Build history of the part. All positions in model axes, mm. A direction names the side the tool comes from. Coordinates: 2 decimals unless noted, no trailing zeros. Loops run counter-clockwise (first coordinate to the right, second up) from the corner with the lowest first, then second, coordinate; pieces in that order, holes last.
(1) Two-plate mould, pull along X, no slides. Class faces 1 (the face through (27.006, -100.787, 9.86)), 2 (the face through (71, 20, 73)), 3 (the face through (29.7, 17, 99.8)), 4 (the face through (97, -34, 20)): pulls with the +X half, pulls with the -X half, needs draft (parallel to the pull), parting line crosses it, or undercut.
(2) Slice it at D-D (x = -12). Give the cut face in (y, z).
(3) Wall check: L1, parallel to Y at x = 30.5, z = 8; L2, parallel to X at y = -66.5, z = 34.5; L3, parallel to Y at x = 60, z = 50. Give the ranges that are in metal, low to high.
(4) Slice it at B-B (z = 66). Give the cut face in (x, y).
(5) Slice it at C-C (y = 4). Give the cut face in (x, z).
(6) Flat gauge pins, fed straight in: P1, Ø4, axis at x = 13.5, y = -91.5, coming from the +Z side; P2, Ø12, axis at y = -99.5, z = 17, coming from the -X side; P3, Ø2, axis at y = -29, z = 31.5, coming from the -X side. Where does each tip first touch, or does it go through?
(7) Slice it at A-A (y = -15). Give the cut face in (x, z).
(8) Tool access for faces 5 (the face through (55.25, -88.42, 4.93)), 6 (the face through (103.73, -10.48, 14.93)), 7 (the face through (26.984, 4.93, 100.705)): list every direction of +Z, -Z, +X, -X, +Y, -Y with a clear straight run to the whole face (end or side of a thin tool).
from build123d import *

# Parameters (mm, degrees)
F1_ANGLE  = 90
F3_DEPTH  = 20
F5_DEPTH  = 20
F7_DEPTH  = 20
F8_R      = 10
F11_DEPTH = 10


with BuildPart() as f1:
    # F0 (on Right) → F1 (revolve)
    with BuildSketch(Plane.YZ):
        with BuildLine():
            Line((0, 94.3), (0, 114.3))
            ThreePointArc((0, 114.3), (-80.8223050896, 80.8223050896), (-114.3, 0))
            Line((-114.3, 0), (-94.3, 0))
            ThreePointArc((-94.3, 0), (-66.6801694659, 66.6801694659), (0, 94.3))
        make_face()
    revolve(axis=Axis((0, 0, 104.3), (0, 0, 1)), revolution_arc=F1_ANGLE)

    # F2 (on face) → F3 (join)
    with BuildSketch(Plane(origin=(0, 0, 0), x_dir=(-1, 0, 0), z_dir=(0, 1, 0))):
        with BuildLine():
            Line((-26.2183692689, 97.8482862031), (-27.7712835395, 103.6438411608))
            ThreePointArc((-27.7712835395, 103.6438411608), (-75.8725576213, 75.8725576213), (-103.6438411608, 27.7712835395))
            Line((-103.6438411608, 27.7712835395), (-97.8482862031, 26.2183692689))
            ThreePointArc((-97.8482862031, 26.2183692689), (-71.6299169342, 71.6299169342), (-26.2183692689, 97.8482862031))
        make_face()
    extrude(amount=F3_DEPTH)

    # F4 (on face) → F5 (join)
    with BuildSketch(Plane.YZ):
        with BuildLine():
            ThreePointArc((-97.8482862031, 26.2183692689), (-71.6299169342, 71.6299169342), (-26.2183692689, 97.8482862031))
            Line((-26.2183692689, 97.8482862031), (-27.7712835395, 103.6438411608))
            ThreePointArc((-27.7712835395, 103.6438411608), (-75.8725576213, 75.8725576213), (-103.6438411608, 27.7712835395))
            Line((-103.6438411608, 27.7712835395), (-97.8482862031, 26.2183692689))
        make_face()
    extrude(amount=-F5_DEPTH)

    # F6 (on face) → F7 (cut)
    with BuildSketch(Plane(origin=(0, 0, 0), x_dir=(1, 0, 0), z_dir=(0, 0, -1))):
        with BuildLine():
            Line((27.7712835395, 103.6438411608), (26.2183692689, 97.8482862031))
            ThreePointArc((26.2183692689, 97.8482862031), (40.3932806821, 92.8981855352), (53.6808214668, 85.9072721406))
            Line((53.6808214668, 85.9072721406), (56.8603370522, 90.9955607176))
            ThreePointArc((56.8603370522, 90.9955607176), (42.7857750957, 98.4005459815), (27.7712835395, 103.6438411608))
        make_face()
        with BuildLine():
            ThreePointArc((84.9573285329, 55.171934247), (92.1790767398, 42.0084254811), (97.3758097986, 27.9220641443))
            Line((97.3758097986, 27.9220641443), (103.1433799742, 29.5758882792))
            ThreePointArc((103.1433799742, 29.5758882792), (97.6388443651, 44.496584937), (89.9893519405, 58.4397684571))
            Line((89.9893519405, 58.4397684571), (84.9573285329, 55.171934247))
        make_face()
    extrude(amount=-F7_DEPTH, mode=Mode.SUBTRACT)

    # F8
    f8_edges = [f1.edges().sort_by_distance(p)[0] for p in [
        (100.746064, 20, 26.994826),
        (26.994826, 20, 100.746064),
        (-20, -26.994826, 100.746064),
        (-20, -100.746064, 26.994826),
    ]]
    fillet(f8_edges, radius=F8_R)

    # F10 (on offset) → F11 (cut)
    with BuildSketch(Plane(origin=(0, 0, 10), x_dir=(1, 0, 0), z_dir=(0, 0, -1))):
        with BuildLine():
            ThreePointArc((97.3758097986, 27.9220641443), (99.4762319066, 19.1355503099), (100.7854867979, 10.1968451452))
            Line((100.7854867979, 10.1968451452), (106.7579299629, 10.7719260129))
            ThreePointArc((106.7579299629, 10.7719260129), (105.3709505868, 20.2546975401), (103.1433799742, 29.5758882792))
            Line((103.1433799742, 29.5758882792), (97.3758097986, 27.9220641443))
        make_face()
        Polygon((0.327321584, 0.5238240331), (0, 0), (0.4947707785, 0.5399475566), align=None)
        Polygon((0.4947707785, 0.5399475566), (0, 0), (2.5848787999, 0.7412020686), align=None)
        with BuildLine():
            Line((56.8603370522, 90.9955607176), (53.6808214668, 85.9072721406))
            ThreePointArc((53.6808214668, 85.9072721406), (61.3162809887, 80.6350028568), (68.4372880315, 74.6861942189))
            Line((68.4372880315, 74.6861942189), (72.4908292772, 79.1098582397))
            ThreePointArc((72.4908292772, 79.1098582397), (64.948044917, 85.411014872), (56.8603370522, 90.9955607176))
        make_face()
    extrude(amount=-F11_DEPTH, mode=Mode.SUBTRACT)


solid = f1.part
Response values:
1. face 1: undercut
1. face 2: needs draft
1. face 3: pulls with the -X half
1. face 4: undercut
2. outline: (-103.59, 27.97) - (-97.8, 26.41) arc R101.3 cw to (-26.41, 97.8) - (-27.97, 103.59) arc R107.3 ccw to start
3. L1: y = -109.86 to -102.87, -96.6 to -88.87
3. L2: x = 57.27 to 86.32
3. L3: y = -83.45 to -52.84
4. outline: (-20, -84.6) - (0, -84.6) - (0, -93.32) arc R93.32 ccw to (93.32, 0) - (84.6, 0) - (84.6, 20) - (76.85, 20) - (76.85, 0) - (67.35, 0) arc R67.35 cw to (0, -67.35) - (0, -76.85) - (-20, -76.85) - close
5. outline: (26.22, 97.85) arc R101.3 cw to (97.85, 26.22) - (103.64, 27.77) arc R107.3 ccw to (27.77, 103.64) - close
6. P1: stops at z = 69.83
6. P2: stops at x = 0
6. P3: stops at x = 83.5
7. outline: (0, 93.1) arc R93.1 cw to (93.1, 0) - (113.31, 0) arc R113.31 ccw to (0, 113.31) - close; hole (100.18, 10) - (106.25, 10) - (106.25, 20) - (100.18, 20) - close
8. face 5: -Z
8. face 6: none
8. face 7: +Z, -X, +Y
